from build123d import *

# Parameters (mm, degrees)
SKETCH1_R           = 10
BOSS_EXTRUDE1_DEPTH = 5.8
BOSS_EXTRUDE2_DEPTH = 5.8
CIRPATTERN1_COUNT   = 24
SKETCH3_R           = 12.65
SKETCH3_R_2         = 12
CUT_EXTRUDE1_DEPTH  = 6
CUT_EXTRUDE2_DEPTH  = 6
SKETCH5_R           = 1.5
CUT_EXTRUDE3_DEPTH  = 6
BOSS_EXTRUDE3_DEPTH = 5.8


with BuildPart() as part:
    # Sketch1 → Boss-Extrude1 (new body)
    with BuildSketch(Plane.XY):
        Circle(SKETCH1_R)
    extrude(amount=BOSS_EXTRUDE1_DEPTH)

    # Sketch2 → Boss-Extrude2 (add)
    with BuildSketch(Plane.XY):
        with BuildLine():
            Line((0, 12.65), (-0.9, 9.959417654))
            ThreePointArc((-0.9, 9.959417654), (0, 10), (0.9, 9.959417654))
            Line((0.9, 9.959417654), (0, 12.65))
        make_face()
    boss_extrude2 = extrude(amount=BOSS_EXTRUDE2_DEPTH)

    # CirPattern1: Boss-Extrude2 ×24 about axis
    cirpattern1_axis = Axis((0, 0, 0), (0, 0, 1))
    for i in range(1, CIRPATTERN1_COUNT):
        add(boss_extrude2.rotate(cirpattern1_axis, i * 360 / CIRPATTERN1_COUNT))

    # Sketch3 → Cut-Extrude1 (cut)
    with BuildSketch(Plane.XY):
        Circle(SKETCH3_R)
        Circle(SKETCH3_R_2, mode=Mode.SUBTRACT)
    extrude(amount=CUT_EXTRUDE1_DEPTH, mode=Mode.SUBTRACT)

    # Sketch4 → Cut-Extrude2 (cut)
    with BuildSketch(Plane.XY):
        with BuildLine():
            Line((0, 0), (0, 12))
            ThreePointArc((0, 12), (11.769423365, -2.341083864), (-4.592201188, -11.08655439))
            Line((-4.592201188, -11.08655439), (-3.826834324, -9.238795325))
            Line((-3.826834324, -9.238795325), (0, 0))
        make_face()
    extrude(amount=CUT_EXTRUDE2_DEPTH, mode=Mode.SUBTRACT)

    # Sketch5 → Cut-Extrude3 (cut)
    with BuildSketch(Plane.XY):
        Circle(SKETCH5_R)
    extrude(amount=CUT_EXTRUDE3_DEPTH, mode=Mode.SUBTRACT)

    # Sketch6 → Boss-Extrude3 (add)
    with BuildSketch(Plane.XY):
        with BuildLine():
            Line((0, 1.5), (0, 12))
            Line((0, 12), (7, 12))
            Line((7, 12), (7, 9.904493766))
            Line((7, 9.904493766), (11, 9.904493766))
            Line((11, 9.904493766), (11, -10.095506234))
            Line((11, -10.095506234), (7, -10.095506234))
            Line((7, -10.095506234), (7, -13.095506234))
            Line((7, -13.095506234), (0, -13.095506234))
            Line((0, -13.095506234), (0, -10.095506234))
            Line((0, -10.095506234), (-3.826834324, -10.095506234))
            Line((-3.826834324, -10.095506234), (-3.826834324, -9.238795325))
            Line((-3.826834324, -9.238795325), (-0.574025149, -1.385819299))
            ThreePointArc((-0.574025149, -1.385819299), (1.471177921, -0.292635483), (0, 1.5))
        make_face()
    extrude(amount=BOSS_EXTRUDE3_DEPTH)


solid = part.part
Design review of the part built by this model. Coordinates are the model's own, in mm. A direction names the side the tool comes from. Give positions to 0.01 mm unless a question says otherwise; leave off trailing zeros. Order: outer loops, then holes, each group sorted by start corner. A loop starts at its lowest first (then second) coordinate and runs counter-clockwise, first axis right, second up.
1. Add section A-A, the plane y = -11.5. State the section outline as (x, z) points.
Solution:
outline: (0, 0) - (7, 0) - (7, 5.8) - (0, 5.8) - close
2. Tool access review of faces 1 (the flat face through (-2, -10.096, 3)), 2 (the cylindrical face through (-9.915, -1.3, 2.859)), 3 (the flat face through (-7.35, 8.15, 2.86)): name each direction out of +Z, -Z, +X, -X, +Y, -Y from which nothing blocks a thin tool from reaching the whole face with its end or side.
Solution:
face 1: +Z, -Z, -Y
face 2: +Z, -Z, -X
face 3: +Z, -Z, +Y
3. For pin 1 Ø1 at (y, z) = (10.5, 4) entering from +X; pin 2 Ø1.9 at (x, z) = (-1.5, 3.5) entering from -Y; pin 3 Ø3 at (y, z) = (5.5, 2.5) entering from -X; pin 4 Ø1.8 at (x, y) = (0, 0) entering from +Z, all flat-tipped, find the tip position at first contact; note any pin that passes through.
Solution:
pin 1: stops at x = 7
pin 2: stops at y = -10.1
pin 3: stops at x = -10.5
pin 4: passes through
4. Add section B-B, the plane y = -2.5. State the section outline as (x, z) points, then the cut area to 3 significant figures.
Solution:
outline: (-11.05, 0) - (11, 0) - (11, 5.8) - (-11.05, 5.8) - close
area: 128 mm2
5. To check wall thickness, follow L1, parallel to X at y = 0, z = 1.45; L2, parallel to Y at x = -8.5, z = 5.45; L3, parallel to Y at x = 8.5, z = 2.05. State the ranges of each line that lie inside material, in increasing order.
Solution:
L1: x = -12 to -1.5, 1.5 to 11
L2: y = -8.47 to -8.05, -5.83 to 5.83, 8.05 to 8.47
L3: y = -10.1 to 9.9
6. Mouldability with a two-part tool opening along X and no side actions: class faces 4 (the flat face through (-8.165, 7.381, 2.859)), 5 (the flat face through (-5.97, -9.21, 2.86)), 6 (the flat face through (2, 0, 5.8)) as +X half, -X half, draft (parallel to the pull), parting line (faces both ways), or undercut.
Solution:
face 4: -X half
face 5: undercut
face 6: draft
